For this review, use the dimensioned drawing (mm, ordinates from the lowest corner) and the shaded views. A direction names the side the tool comes from. Coordinates: 2 decimals unless noted, no trailing zeros. Order: outer loops, then holes, each group sorted by start corner. A loop starts at its lowest first (then second) coordinate and runs counter-clockwise, first axis right, second up. Notation, with made-up numbers: M -20.75,74 L -14.75,74 A31 cw -14.75,100 Z; hole C -9,17 d5. An arc over 180 degrees is marked long. Use one line per item in the form item = value. Start each with the question number.
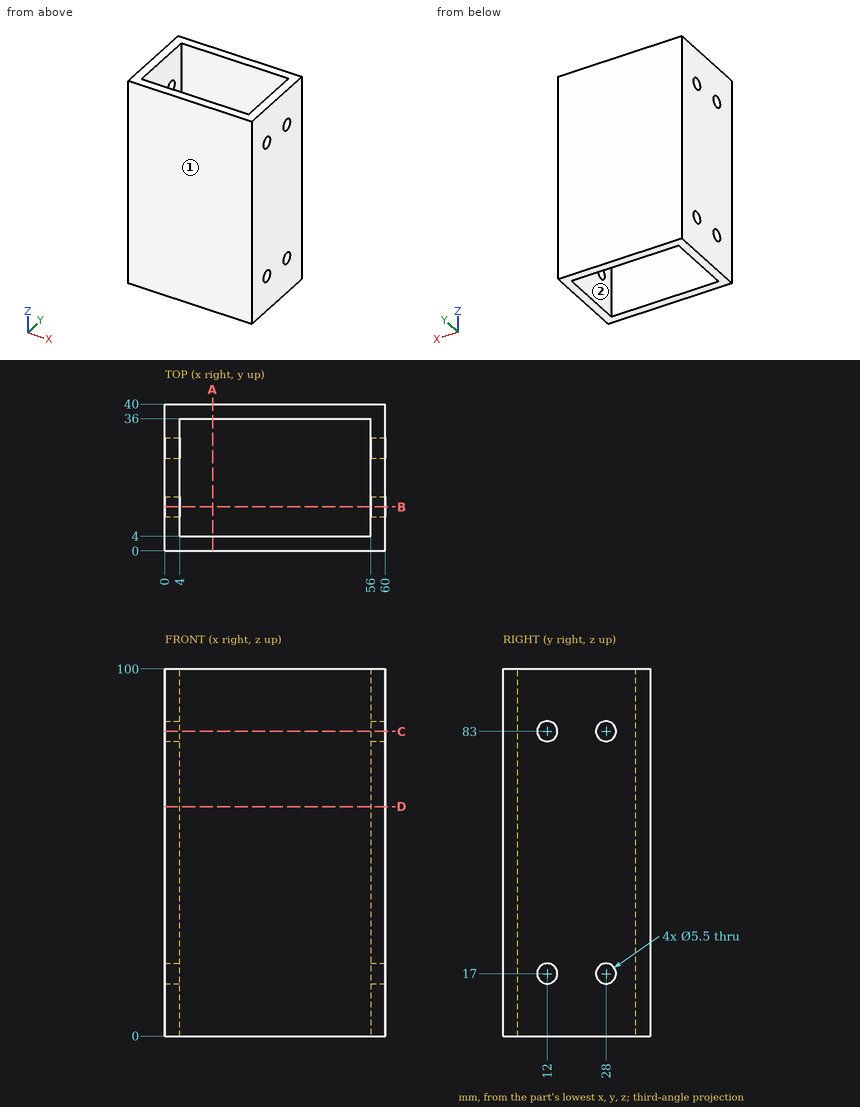
1. Tool access review of the marked faces 1 and 2: name each direction out of +Z, -Z, +X, -X, +Y, -Y from which nothing blocks a thin tool from reaching the whole face with its end or side.
2. Consider section D-D, the plane z = 62.5. Write out the cut boundary in (x, y).
3. Consider section B-B, the plane y = 12. Write out the cut boundary in (x, z).
4. To check wall thickness, follow line 1 (Y direction, x = 57, z = 17); line 2 (X direction, y = 14, z = 90.5); line 3 (Y direction, x = 54.5, z = 22). State the ranges of each line that lie inside material, in increasing order.
5. Consider section A-A, the plane x = 13. Write out the cut boundary in (y, z).
6. Consider section C-C, the plane z = 83. Write out the cut boundary in (x, y), plus the area to 3 significant figures.
Answers follow:
q1.face_1 = +Z, -Z, +X, -X, -Y
q1.face_2 = +Z, -Z
q2.outline = M 0,0 L 60,0 L 60,40 L 0,40 Z; hole M 4,4 L 56,4 L 56,36 L 4,36 Z
q3.outline = M 0,0 L 4,0 L 4,14.25 L 0,14.25 Z; M 0,19.75 L 4,19.75 L 4,80.25 L 0,80.25 Z; M 0,85.75 L 4,85.75 L 4,100 L 0,100 Z; M 56,0 L 60,0 L 60,14.25 L 56,14.25 Z; M 56,19.75 L 60,19.75 L 60,80.25 L 56,80.25 Z; M 56,85.75 L 60,85.75 L 60,100 L 56,100 Z
q4.line_1 = 0 to 9.25, 14.75 to 25.25, 30.75 to 40
q4.line_2 = 0 to 4, 56 to 60
q4.line_3 = 0 to 4, 36 to 40
q5.outline = M 0,0 L 4,0 L 4,100 L 0,100 Z; M 36,0 L 40,0 L 40,100 L 36,100 Z
q6.outline = M 0,0 L 60,0 L 60,9.25 L 56,9.25 L 56,4 L 4,4 L 4,9.25 L 0,9.25 Z; M 0,14.75 L 4,14.75 L 4,25.25 L 0,25.25 Z; M 0,30.75 L 4,30.75 L 4,36 L 56,36 L 56,30.75 L 60,30.75 L 60,40 L 0,40 Z; M 56,14.75 L 60,14.75 L 60,25.25 L 56,25.25 Z
q6.area = 648 mm²
